Build history of the part. All positions in model axes, mm. A direction names the side the tool comes from. Round coordinates to 2 decimals unless told otherwise and drop trailing zeros. Write each loop counter-clockwise with the first axis right and the second up, starting at its lowest first coordinate (ties: lowest second). Pieces come first, ordered by that corner, then holes.
1) Flat gauge pins, fed straight in: pin 1 (2.5 mm diameter, centred on y = 26, z = 15, fed in from -X); pin 2 (2.5 mm diameter, centred on y = 6, z = 15, fed in from +X). Where does each tip first touch, or does it go through?
2) Saw through at A-A (z = 18.5). Write the cut outline in (x, y), plus the area to 3 significant figures.
3) Pull direction Y, two halves, no side cores. Call faces 1 (the cylindrical face through (-3.45, 5.93, 3.35)), 2 (the flat face through (-13, 0, 10)), 3 (the flat face through (-13, 32, 10)): +Y half, -Y half, draft (parallel to the pull), parting line (faces both ways), or undercut.
4) Saw through at B-B (x = -23). Write the cut outline in (y, z).
5) Saw through at C-C (x = -12.5). Write the cut outline in (y, z), plus the area to 3 significant figures.
6) Wall check: probe 1 along Z at (x, y) = (-20, 6); probe 2 along Y at (x, z) = (-20.25, 15); probe 3 along Y at (x, z) = (-1.5, 16). Give the ranges that are in metal, low to high.
7) Which spindle directions (+Z, -Z, +X, -X, +Y, -Y) get a long thin tool onto all of the face, cutting with end or side? Do faces 4 (the flat face through (0, 16, 10)), 5 (the cylindrical face through (-3.45, 24.61, 15.89)), 6 (the cylindrical face through (-21.55, 24.61, 15.89)), 7 (the flat face through (-18.2, 12.7, 0)), 8 (the flat face through (-14.088, 23, 10)). Say none if no direction does.
8) Saw through at D-D (y = 19). Write the cut outline in (x, z), plus the area to 3 significant figures.
from build123d import *

# Parameters (mm, degrees)
SKETCH1_W                      = 25
SKETCH1_H                      = 32
BOSS_EXTRUDE1_DEPTH            = 20
CUT_EXTRUDE1_DEPTH             = 21
M4X0_7_TAPPED_HOLE1_AT_2_COUNT = 2
M4X0_7_TAPPED_HOLE1_AT_2_PITCH = 22.360679775
M4X0_7_TAPPED_HOLE1_AT_3_COUNT = 2
M4X0_7_TAPPED_HOLE1_AT_3_PITCH = 20
M4X0_7_TAPPED_HOLE1_AT_4_COUNT = 2
M4X0_7_TAPPED_HOLE1_AT_4_PITCH = 10
FILLET1_R                      = 0.5


with BuildPart() as part:
    # Sketch1 → Boss-Extrude1 (new body)
    with BuildSketch(Plane.XY):
        with Locations((-12.5, 16)):
            Rectangle(SKETCH1_W, SKETCH1_H)
    extrude(amount=BOSS_EXTRUDE1_DEPTH)

    # Sketch2 → Cut-Extrude1 (cut, through all)
    with BuildSketch(Plane.XY.offset(20)):
        with BuildLine():
            ThreePointArc((-10.9125, 22.148361062), (-12.5, 22.35), (-14.0875, 22.148361062))
            Line((-14.0875, 22.148361062), (-14.0875, 20.7625))
            Line((-14.0875, 20.7625), (-10.9125, 20.7625))
            Line((-10.9125, 20.7625), (-10.9125, 22.148361062))
        make_face()
        with BuildLine():
            Line((-14.0875, 20.7625), (-14.0875, 22.148361062))
            ThreePointArc((-14.0875, 22.148361062), (-16.388564967, 10.979884214), (-6.15, 16))
            ThreePointArc((-6.15, 16), (-7.479884214, 19.888564967), (-10.9125, 22.148361062))
            Line((-10.9125, 22.148361062), (-10.9125, 20.7625))
            Line((-10.9125, 20.7625), (-14.0875, 20.7625))
        make_face()
        with BuildLine():
            Line((-10.9125, 24.4625), (-14.0875, 24.4625))
            Line((-14.0875, 24.4625), (-14.0875, 22.148361062))
            ThreePointArc((-14.0875, 22.148361062), (-12.5, 22.35), (-10.9125, 22.148361062))
            Line((-10.9125, 22.148361062), (-10.9125, 24.4625))
        make_face()
    extrude(amount=-CUT_EXTRUDE1_DEPTH, mode=Mode.SUBTRACT)

    # Sketch4 → M4x0.7 Tapped Hole1 (revolve, cut)
    with BuildSketch(Plane(origin=(-25, 26, 5), x_dir=(0, 0, 1), z_dir=(0, 1, 0))):
        Polygon((0, 0), (0, 7.991420021), (1.65, 7), (1.65, 0), align=None)
    m4x0_7_tapped_hole1 = revolve(axis=Axis((-31.35, 26, 5), (1, 0, 0)), mode=Mode.SUBTRACT)

    # M4x0.7 Tapped Hole1 at 2: M4x0.7 Tapped Hole1 ×2
    with Locations(*[Vector(0, -0.894427191, 0.447213595) * (i * M4X0_7_TAPPED_HOLE1_AT_2_PITCH) for i in range(1, M4X0_7_TAPPED_HOLE1_AT_2_COUNT)]):
        add(m4x0_7_tapped_hole1, mode=Mode.SUBTRACT)

    # M4x0.7 Tapped Hole1 at 3: M4x0.7 Tapped Hole1 ×2
    with Locations(*[(0, -i * M4X0_7_TAPPED_HOLE1_AT_3_PITCH, 0) for i in range(1, M4X0_7_TAPPED_HOLE1_AT_3_COUNT)]):
        add(m4x0_7_tapped_hole1, mode=Mode.SUBTRACT)

    # M4x0.7 Tapped Hole1 at 4: M4x0.7 Tapped Hole1 ×2
    with Locations(*[(0, 0, i * M4X0_7_TAPPED_HOLE1_AT_4_PITCH) for i in range(1, M4X0_7_TAPPED_HOLE1_AT_4_COUNT)]):
        add(m4x0_7_tapped_hole1, mode=Mode.SUBTRACT)

    # Mirror1: M4x0.7 Tapped Hole1 across plane
    add(m4x0_7_tapped_hole1.mirror(Plane.ZY.offset(12.5)), mode=Mode.SUBTRACT)

    # Mirror1 copy 1 sketch → Mirror1 copy 1 (revolve, cut)
    with BuildSketch(Plane(origin=(0, 6, 15), x_dir=(0, 0, 1), z_dir=(0, 1, 0))):
        Polygon((0, 0), (0, -7.991420021), (1.65, -7), (1.65, 0), align=None)
    revolve(axis=Axis((6.35, 6, 15), (1, 0, 0)), mode=Mode.SUBTRACT)

    # Mirror1 copy 2 sketch → Mirror1 copy 2 (revolve, cut)
    with BuildSketch(Plane(origin=(0, 6, 5), x_dir=(0, 0, 1), z_dir=(0, 1, 0))):
        Polygon((0, 0), (0, -7.991420021), (1.65, -7), (1.65, 0), align=None)
    revolve(axis=Axis((6.35, 6, 5), (1, 0, 0)), mode=Mode.SUBTRACT)

    # Mirror1 copy 3 sketch → Mirror1 copy 3 (revolve, cut)
    with BuildSketch(Plane(origin=(0, 26, 15), x_dir=(0, 0, 1), z_dir=(0, 1, 0))):
        Polygon((0, 0), (0, -7.991420021), (1.65, -7), (1.65, 0), align=None)
    revolve(axis=Axis((6.35, 26, 15), (1, 0, 0)), mode=Mode.SUBTRACT)

    # Fillet1
    fillet1_edges = [part.edges().sort_by_distance(p)[0] for p in [
        (-14.0875, 24.4625, 10),
        (-10.9125, 24.4625, 10),
    ]]
    fillet(fillet1_edges, radius=FILLET1_R)


solid = part.part
Evaluation:
1. pin 1: stops at x = -17.76
1. pin 2: stops at x = -7.24
2. outline: (-25, 0) - (0, 0) - (0, 32) - (-25, 32) - close; hole (-14.09, 22.15) arc R6.35 ccw (long way) to (-10.91, 22.15) - (-10.91, 23.96) arc R0.5 ccw to (-11.41, 24.46) - (-13.59, 24.46) arc R0.5 ccw to (-14.09, 23.96) - close
2. area: 667 mm2
3. face 1: undercut
3. face 2: -Y half
3. face 3: +Y half
4. outline: (0, 0) - (32, 0) - (32, 20) - (0, 20) - close; hole circle Ø3.3 at (6, 5); hole circle Ø3.3 at (6, 15); hole circle Ø3.3 at (26, 5); hole circle Ø3.3 at (26, 15)
5. outline: (0, 0) - (9.65, 0) - (9.65, 20) - (0, 20) - close; (24.46, 0) - (32, 0) - (32, 20) - (24.46, 20) - close
5. area: 344 mm2
6. probe 1: z = 0 to 3.35, 6.65 to 13.35, 16.65 to 20
6. probe 2: y = 0 to 4.35, 7.65 to 24.35, 27.65 to 32
6. probe 3: y = 0 to 4.69, 7.31 to 24.69, 27.31 to 32
7. face 4: +Z, -Z, +X, +Y, -Y
7. face 5: +X
7. face 6: -X
7. face 7: -Z, +X, -X, +Y, -Y
7. face 8: +Z, -Z
8. outline: (-25, 0) - (-18.1, 0) - (-18.1, 20) - (-25, 20) - close; (-6.9, 0) - (0, 0) - (0, 20) - (-6.9, 20) - close
8. area: 276 mm2
